Autodesk Inventor part; units mm, degrees
ref_plane "YZ Plane" through (0, 0, 0) normal (1, 0, 0) x (0, 1, 0)
ref_plane "XZ Plane" through (0, 0, 0) normal (0, 1, 0) x (-1, 0, 0)
ref_plane "XY Plane" through (0, 0, 0) normal (0, 0, 1) x (1, 0, 0)
sketch "Skizze1" plane through (0, 0, 0) normal (0, 1, 0) x (-1, 0, 0)
  circle A0 centre (0, 0) radius 14
  dimension "d0" = 28
extrude "Extrusion1" add sketch "Skizze1" along normal blind 51
sketch "Skizze2" plane through (0, 0, 0) normal (0, -1, 0) x (1, 0, 0)
  line L0 (-25, 25) -> (25, 25)
  line L1 (25, 25) -> (25, -25)
  line L2 (25, -25) -> (-25, -25)
  line L3 (-25, -25) -> (-25, 25)
  line L4 (-25, 25) -> (25, -25) construction
  line L5 (25, 25) -> (-25, -25) construction
  point P0 (0, 0)
  dimension "d3" = 50
  dimension "d4" = 50
extrude "Extrusion2" add sketch "Skizze2" along normal mid plane 5
chamfer "Fasen1" distance 1 angle 45 1 edges at (14, 51, 0)
sketch "Skizze3" plane through (0, -2.5, 0) normal (0, -1, 0) x (1, 0, 0)
  point P0 (0, 0)
  point P1 (0, 0)
hole "Bohrung1" at (0, -2.5, 0) direction (0, 1, 0) diameter 27 end through all
sketch "Skizze4" plane through (0, -2.5, 0) normal (0, -1, 0) x (1, 0, 0)
  line L0 (-25, -25) -> (-25, 25)
  line L1 (-25, 0) -> (25, 0) construction
  line L2 (25, 25) -> (25, -25)
  line L3 (-25, 25) -> (25, 25)
  line L4 (0, 25) -> (0, -21.9496) construction
  point P0 (0, 0)
  point P1 (-21.124, -21.124)
  point P2 (-21.124, 21.124)
  point P3 (21.124, -21.124)
  point P4 (21.124, 21.124)
  dimension "d30" = 42.248
  dimension "d31" = 42.248
  dimension "d32" = 42.248
  dimension "d33" = 42.248
hole "Bohrung2" at (-21.124, -2.5, -21.124) at (-21.124, -2.5, 21.124) at (21.124, -2.5, -21.124) at (21.124, -2.5, 21.124) direction (0, 1, 0) diameter 5 depth 5
properties part number "candle_cylinder" material "Gold"
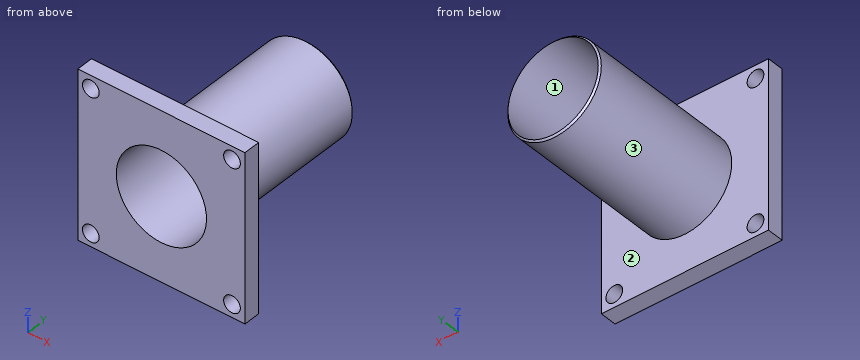
The listing builds one solid part. Answer for the finished solid, in the listing's coordinates (mm). Face numbers are marked on the shaded views. Coordinates: 2 decimals unless noted, no trailing zeros. Write each loop counter-clockwise with the first axis right and the second up, starting at its lowest first coordinate (ties: lowest second). Pieces come first, ordered by that corner, then holes. Notation, with made-up numbers: M 4,31.5 L 41,31.5 A30 ccw 41,69.5 Z; hole C 37,39 d11. An arc over 180 degrees is marked long. Use one line per item in the form item = value.
Item 1: Find the intervals of material crossed by probe 1 along X at (y, z) = (21.5, 0); probe 2 along Z at (x, y) = (-12, 27.5); probe 3 along Z at (x, y) = (-4.5, 35), in increasing order.
Model answer:
probe_1 = -14 to -13.5, 13.5 to 14
probe_2 = -7.21 to -6.18, 6.18 to 7.21
probe_3 = -13.26 to -12.73, 12.73 to 13.26
Item 2: The mould has two halves that part along Z. Classify the marked faces 1, 2 and 3: released by +Z, released by -Z, zero draft, split by the parting line, or undercut.
Model answer:
face_1 = undercut
face_2 = zero draft
face_3 = split by the parting line
Item 3: Find section D-D, the plane y = 18.5. Give the vertices of the cut face in (x, z).
Model answer:
outline = C 0,0 d28; hole C 0,0 d27
Item 4: Given P1, Ø5, axis at x = -1, y = 43.5, coming from the -Z side; P2, Ø16, axis at x = 0, z = 0, coming from the +Y side; P3, Ø1.5, axis at y = 5.5, z = 13, coming from the +X side; P4, Ø12, axis at x = -15, y = 39, coming from the +Z side, each flat-ended and moving along its own axis, determine where each tip first touches the part or whether it passes through.
Model answer:
P1 = -14
P2 = through
P3 = 6.78
P4 = 10.72
Item 5: Find section A-A, the plane x = 0. Give the vertices of the cut face in (y, z).
Model answer:
outline = M -2.5,-25 L 2.5,-25 L 2.5,-14 L 50,-14 L 50.5,-13.5 L -2.5,-13.5 Z; M -2.5,13.5 L 50.5,13.5 L 50,14 L 2.5,14 L 2.5,25 L -2.5,25 Z
Item 6: Find section B-B, the plane z = 0. Give the vertices of the cut face in (x, y), plus the area to 3 significant figures.
Model answer:
outline = M -25,-2.5 L -13.5,-2.5 L -13.5,50.5 L -14,50 L -14,2.5 L -25,2.5 Z; M 13.5,-2.5 L 25,-2.5 L 25,2.5 L 14,2.5 L 14,50 L 13.5,50.5 Z
area = 163 mm2
Item 7: Find section C-C, the plane z = 20.5. Give the vertices of the cut face in (x, y).
Model answer:
outline = M -25,-2.5 L -23.54,-2.5 L -23.54,2.5 L -25,2.5 Z; M -18.7,-2.5 L 18.7,-2.5 L 18.7,2.5 L -18.7,2.5 Z; M 23.54,-2.5 L 25,-2.5 L 25,2.5 L 23.54,2.5 Z
